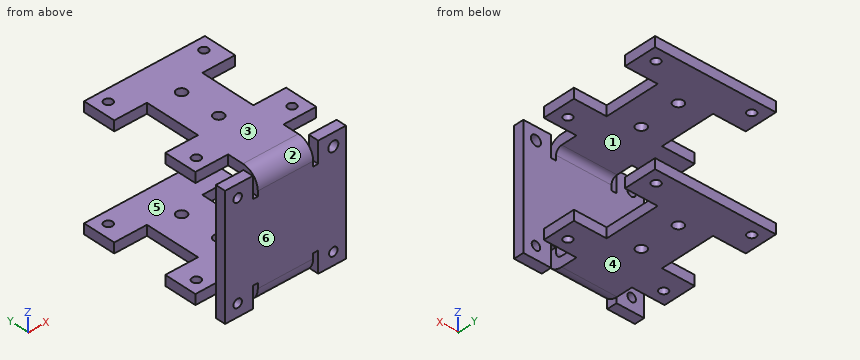
```python
from build123d import *

# Parameters (mm, degrees)
SKETCH_16_R                       = 2.1
SKETCH_16_R_2                     = 2.5
SM_BASE_FLANGE_2_DEPTH            = 5
SM_EDGE_FLANGE_1_STRIP_W          = 26
SM_EDGE_FLANGE_1_STRIP_H          = 5
SM_EDGE_FLANGE_1_STRIP_CUT_DEPTH  = 27.5
SM_EDGE_FLANGE_1_RELIEF_W         = 28.5
SM_EDGE_FLANGE_1_RELIEF_H         = 2.5
SM_EDGE_FLANGE_1_RELIEF_CUT_DEPTH = 5
SM_EDGE_FLANGE_1_DEPTH            = 27.5
SM_EDGE_FLANGE_2_STRIP_W          = 26
SM_EDGE_FLANGE_2_STRIP_H          = 5
SM_EDGE_FLANGE_2_STRIP_CUT_DEPTH  = 27.5
SM_EDGE_FLANGE_2_RELIEF_W         = 28.5
SM_EDGE_FLANGE_2_RELIEF_H         = 2.5
SM_EDGE_FLANGE_2_RELIEF_CUT_DEPTH = 5
SM_EDGE_FLANGE_2_DEPTH            = 27.5
EXTRUDE_START                     = 30
SKETCH_23_W                       = 16.25
SKETCH_23_H                       = 16.25
EXTRUDE_1_DEPTH                   = 5
EXTRUDE_START_2                   = -25
SKETCH_24_W                       = 16.25
SKETCH_24_H                       = 16.25
EXTRUDE_2_DEPTH                   = 5
CUT_EXTRUDE_1_DEPTH               = 83.710337927
CUT_EXTRUDE_1_DEPTH_BACK          = 83.710337927
SKETCH_25_R                       = 2.1
CUT_EXTRUDE_2_DEPTH               = 83.710337927
CUT_EXTRUDE_2_DEPTH_BACK          = 83.710337927
SKETCH_26_R                       = 2.5


# Sheet-metal steps are written as plain solids
with BuildPart() as part:
    # 草图16 → 基体-法兰2 (new body)
    with BuildSketch(Plane(origin=(0, 0, 0), x_dir=(1, 0, 0), z_dir=(0, 1, 0))):
        Polygon((16.25, 30), (30, 30), (30, -30), (16.25, -30), (16.25, -25), (-16.25, -25), (-16.25, -30), (-30, -30), (-30, 30), (-16.25, 30), (-16.25, 25), (16.25, 25), align=None)
        with Locations(Location((-23.75, 23.75, 0), (0, 0, 270))):
            Circle(SKETCH_16_R, mode=Mode.SUBTRACT)
        with Locations(Location((-23.75, -23.75, 0), (0, 0, 270))):
            Circle(SKETCH_16_R, mode=Mode.SUBTRACT)
        with Locations(Location((23.75, 23.75, 0), (0, 0, 270))):
            Circle(SKETCH_16_R, mode=Mode.SUBTRACT)
        with Locations(Location((23.75, -23.75, 0), (0, 0, 270))):
            Circle(SKETCH_16_R_2, mode=Mode.SUBTRACT)
    extrude(amount=-SM_BASE_FLANGE_2_DEPTH)

    # 边线-法兰1 strip (across the edge) → 边线-法兰1 strip cut (cut)
    with BuildSketch(Plane(origin=(-13.75, 0, 25), x_dir=(0, 0, -1), z_dir=(1, 0, 0))):
        with Locations((-10, -2.5)):
            Rectangle(SM_EDGE_FLANGE_1_STRIP_W, SM_EDGE_FLANGE_1_STRIP_H)
    extrude(amount=SM_EDGE_FLANGE_1_STRIP_CUT_DEPTH, mode=Mode.SUBTRACT)

    # 边线-法兰1 relief (on the sheet) → 边线-法兰1 relief cut (cut)
    with BuildSketch(Plane(origin=(-13.75, 0, 22), x_dir=(0, 0, -1), z_dir=(0, 1, 0))):
        with Locations((-11.75, 1.25)):
            Rectangle(SM_EDGE_FLANGE_1_RELIEF_W, SM_EDGE_FLANGE_1_RELIEF_H)
        with Locations((-11.75, -28.75)):
            Rectangle(SM_EDGE_FLANGE_1_RELIEF_W, SM_EDGE_FLANGE_1_RELIEF_H)
    extrude(amount=-SM_EDGE_FLANGE_1_RELIEF_CUT_DEPTH, mode=Mode.SUBTRACT)

    # 边线-法兰1 section (across the edge) → 边线-法兰1 (add)
    with BuildSketch(Plane(origin=(-13.75, 0, 25), x_dir=(0, 0, -1), z_dir=(1, 0, 0))):
        with BuildLine():
            Line((-5, 3), (-5, 71))
            Line((-5, 71), (0, 71))
            Line((0, 71), (0, 3))
            ThreePointArc((0, 3), (0.878679656, 0.878679656), (3, 0))
            Line((3, 0), (3, -5))
            ThreePointArc((3, -5), (-2.656854249, -2.656854249), (-5, 3))
        make_face()
    extrude(amount=SM_EDGE_FLANGE_1_DEPTH)

    # 边线-法兰2 strip (across the edge) → 边线-法兰2 strip cut (cut)
    with BuildSketch(Plane(origin=(13.75, 0, -25), x_dir=(0, 0, 1), z_dir=(-1, 0, 0))):
        with Locations((-10, -2.5)):
            Rectangle(SM_EDGE_FLANGE_2_STRIP_W, SM_EDGE_FLANGE_2_STRIP_H)
    extrude(amount=SM_EDGE_FLANGE_2_STRIP_CUT_DEPTH, mode=Mode.SUBTRACT)

    # 边线-法兰2 relief (on the sheet) → 边线-法兰2 relief cut (cut)
    with BuildSketch(Plane(origin=(13.75, 0, -22), x_dir=(0, 0, 1), z_dir=(0, 1, 0))):
        with Locations((-11.75, 1.25)):
            Rectangle(SM_EDGE_FLANGE_2_RELIEF_W, SM_EDGE_FLANGE_2_RELIEF_H)
        with Locations((-11.75, -28.75)):
            Rectangle(SM_EDGE_FLANGE_2_RELIEF_W, SM_EDGE_FLANGE_2_RELIEF_H)
    extrude(amount=-SM_EDGE_FLANGE_2_RELIEF_CUT_DEPTH, mode=Mode.SUBTRACT)

    # 边线-法兰2 section (across the edge) → 边线-法兰2 (add)
    with BuildSketch(Plane(origin=(13.75, 0, -25), x_dir=(0, 0, 1), z_dir=(-1, 0, 0))):
        with BuildLine():
            Line((-5, 3), (-5, 71))
            Line((-5, 71), (0, 71))
            Line((0, 71), (0, 3))
            ThreePointArc((0, 3), (0.878679656, 0.878679656), (3, 0))
            Line((3, 0), (3, -5))
            ThreePointArc((3, -5), (-2.656854249, -2.656854249), (-5, 3))
        make_face()
    extrude(amount=SM_EDGE_FLANGE_2_DEPTH)

    # 草图23 → 凸台-拉伸1 (add)
    with BuildSketch(Plane.XY.offset(EXTRUDE_START)):
        with Locations((-21.875, 62.875)):
            Rectangle(SKETCH_23_W, SKETCH_23_H)
        with Locations((21.875, 62.875)):
            Rectangle(SKETCH_23_W, SKETCH_23_H)
        with Locations((21.875, 19.125)):
            Rectangle(SKETCH_23_W, SKETCH_23_H)
        with Locations((-21.875, 19.125)):
            Rectangle(SKETCH_23_W, SKETCH_23_H)
    extrude(amount=-EXTRUDE_1_DEPTH)

    # 草图24 → 凸台-拉伸2 (add)
    with BuildSketch(Plane.XY.offset(EXTRUDE_START_2)):
        with Locations((21.875, 62.875)):
            Rectangle(SKETCH_24_W, SKETCH_24_H)
        with Locations((-21.875, 62.875)):
            Rectangle(SKETCH_24_W, SKETCH_24_H)
        with Locations((-21.875, 19.125)):
            Rectangle(SKETCH_24_W, SKETCH_24_H)
        with Locations((21.875, 19.125)):
            Rectangle(SKETCH_24_W, SKETCH_24_H)
    extrude(amount=-EXTRUDE_2_DEPTH)

    # 草图25 → 切除-拉伸1 (cut, two sides: drawn at the far end of the back side and taken through both)
    with BuildSketch(Plane.XY.offset(-CUT_EXTRUDE_1_DEPTH_BACK)):
        with Locations((-23.75, 64.75)):
            Circle(SKETCH_25_R)
        with Locations((23.75, 64.75)):
            Circle(SKETCH_25_R)
        with Locations((-23.75, 17.25)):
            Circle(SKETCH_25_R)
        with Locations((23.75, 17.25)):
            Circle(SKETCH_25_R)
    extrude(amount=CUT_EXTRUDE_1_DEPTH + CUT_EXTRUDE_1_DEPTH_BACK, mode=Mode.SUBTRACT)

    # 草图26 → 切除-拉伸2 (cut, two sides: drawn at the far end of the back side and taken through both)
    with BuildSketch(Plane.XY.offset(-CUT_EXTRUDE_2_DEPTH_BACK)):
        with Locations((0, 51)):
            Circle(SKETCH_26_R)
        with Locations((0, 31)):
            Circle(SKETCH_26_R)
    extrude(amount=CUT_EXTRUDE_2_DEPTH + CUT_EXTRUDE_2_DEPTH_BACK, mode=Mode.SUBTRACT)


solid = part.part
```
Design review of the part built by this model. Coordinates are the model's own, in mm. Face numbers are marked on the shaded views. A direction names the side the tool comes from. Round coordinates to 2 decimals unless told otherwise and drop trailing zeros. Write each loop counter-clockwise with the first axis right and the second up, starting at its lowest first coordinate (ties: lowest second). Pieces come first, ordered by that corner, then holes.
Item 1: For the marked faces 1, 2 and 3, list the 3-axis set-ups (+Z, -Z, +X, -X, +Y, -Y) from which the entire face can be reached by the end or side of a thin tool; tool diameter is ignored.
Item 2: For probe 1 along Y at (x, z) = (-23.75, 28.9); probe 2 along X at (y, z) = (-3.5, -23.75); probe 3 along Z at (x, y) = (11, 39), list the stretches that pass through material, from the lowest coordinate up.
Item 3: We need section B-B on x = 0. Write out the cut boundary in (y, z).
Item 4: The part is to be moulded in two halves that separate along Z. For the marked faces 4, 5 and 6, say which applies: +Z half, -Z half, draft (parallel to the pull), parting line (faces both ways), or undercut.
Item 5: Clearance check with flat-ended pins moving along their axes: pin 1 Ø4 at (x, z) = (-23.75, -23.75) entering from +Y; pin 2 Ø2 at (x, y) = (14.5, -3) entering from -Z; pin 3 Ø10 at (x, z) = (14.5, -5) entering from +Y; pin 4 Ø3 at (x, z) = (23.75, 23.75) entering from -Y. State where each tip first meets the part, or that it passes through.
Item 6: We need section D-D on z = -23.75. Write out the cut boundary in (x, y).
Item 7: We need section C-C on y = 35.5. Write out the cut boundary in (x, z).
Item 8: We need section A-A on y = 51. Write out the cut boundary in (x, z), and give its area (3 significant figures).
Returned:
1. face 1: +X, -X, +Y
1. face 2: +Z, -Y
1. face 3: +Z, +X, -X, +Y, -Y
2. probe 1: y = -5 to 0, 11 to 15.15, 19.35 to 27.25, 54.75 to 62.65, 66.85 to 71
2. probe 2: x = -30 to -25.85, -21.65 to -16.25, -13.75 to 13.75, 16.25 to 21.65, 25.85 to 30
2. probe 3: z = -30 to -25, 25 to 30
3. outline: (-5, -22) arc R8 ccw to (3, -30) - (28.5, -30) - (28.5, -25) - (3, -25) arc R3 cw to (0, -22) - (0, 22) arc R3 cw to (3, 25) - (28.5, 25) - (28.5, 30) - (3, 30) arc R8 ccw to (-5, 22) - close; (33.5, -30) - (48.5, -30) - (48.5, -25) - (33.5, -25) - close; (33.5, 25) - (48.5, 25) - (48.5, 30) - (33.5, 30) - close; (53.5, -30) - (71, -30) - (71, -25) - (53.5, -25) - close; (53.5, 25) - (71, 25) - (71, 30) - (53.5, 30) - close
4. face 4: -Z half
4. face 5: undercut
4. face 6: draft
5. pin 1: stops at y = 71
5. pin 2: stops at z = -27.96
5. pin 3: stops at y = 0
5. pin 4: stops at y = 11
6. outline: (-30, -5) - (-25.85, -5) - (-25.85, 0) - (-30, 0) - close; (-21.65, -5) - (-16.25, -5) - (-16.25, 0) - (-21.65, 0) - close; (-13.75, -4.81) - (13.75, -4.81) - (13.75, 0.56) - (-13.75, 0.56) - close; (16.25, -5) - (21.65, -5) - (21.65, 0) - (16.25, 0) - close; (25.85, -5) - (30, -5) - (30, 0) - (25.85, 0) - close
7. outline: (-13.75, -30) - (13.75, -30) - (13.75, -25) - (-13.75, -25) - close; (-13.75, 25) - (13.75, 25) - (13.75, 30) - (-13.75, 30) - close
8. outline: (-13.75, -30) - (-2.5, -30) - (-2.5, -25) - (-13.75, -25) - close; (-13.75, 25) - (-2.5, 25) - (-2.5, 30) - (-13.75, 30) - close; (2.5, -30) - (13.75, -30) - (13.75, -25) - (2.5, -25) - close; (2.5, 25) - (13.75, 25) - (13.75, 30) - (2.5, 30) - close
8. area: 225 mm2
